Design review of the part built by this model. Coordinates are the model's own, in mm. Give positions to 0.01 mm unless a question says otherwise; leave off trailing zeros. Order: outer loops, then holes, each group sorted by start corner. A loop starts at its lowest first (then second) coordinate and runs counter-clockwise, first axis right, second up. Notation, with made-up numbers: (23, 55) -> (54, 55) arc R31 ccw to (54, 86) -> close; hole circle Ø8 at (3.25, 18). An arc over 180 degrees is marked (long way). Answer in a Markdown table with one row per item. Add a question column.
```python
from build123d import *

# Parameters (mm, degrees)
F0_R     = 10.9982
F1_DEPTH = 6.35


with BuildPart() as f1:
    # F0 (on Front) → F1 (new body)
    with BuildSketch(Plane.XZ):
        with BuildLine():
            ThreePointArc((12.7012721412, 6.542961275), (13.8852814514, 3.3662464655), (14.2875, 0))
            ThreePointArc((14.2875, 0), (9.8578957303, -10.3418831951), (-0.6842652522, -14.2711049788))
            ThreePointArc((-0.6842652522, -14.2711049788), (7.240663618, -16.8071465228), (12.8358325851, -22.965887347))
            ThreePointArc((12.8358325851, -22.965887347), (13.5200979128, -8.6947823719), (26.2213700252, -2.151821041))
            ThreePointArc((26.2213700252, -2.151821041), (18.2964411378, 0.3842204693), (12.7012721412, 6.542961275))
        make_face()
        with BuildLine():
            ThreePointArc((-14.9742166985, -21.6324620433), (-8.8154758203, -16.0372930271), (-0.6842652522, -14.2711049788))
            ThreePointArc((-0.6842652522, -14.2711049788), (-12.7012721174, -6.5429613211), (-12.0170067319, 7.7281437263))
            ThreePointArc((-12.0170067319, 7.7281437263), (-18.1757475859, 2.1329746676), (-26.3069581555, 0.366786576))
            ThreePointArc((-26.3069581555, 0.366786576), (-16.649340262, -4.0464226961), (-12.7037234832, -13.9043183991))
            ThreePointArc((-12.7037234832, -13.9043183991), (-13.283093766, -17.9317041401), (-14.9742166985, -21.6324620433))
        make_face()
        with BuildLine():
            ThreePointArc((-12.0170067319, 7.7281437263), (0.6842654078, 14.2711049713), (12.7012721412, 6.542961275))
            ThreePointArc((12.7012721412, 6.542961275), (10.9350840416, 14.6741718257), (13.4711255704, 22.5991007709))
            ThreePointArc((13.4711255704, 22.5991007709), (0.769853458, 16.0561394401), (-11.2471533267, 23.7842830843))
            ThreePointArc((-11.2471533267, 23.7842830843), (-9.4809652551, 15.6530726068), (-12.0170067319, 7.7281437263))
        make_face()
        with BuildLine():
            ThreePointArc((39.8246046975, -16.4229260161), (35.8789879186, -6.5650303131), (26.2213700252, -2.151821041))
            ThreePointArc((26.2213700252, -2.151821041), (13.5200979128, -8.6947823719), (12.8358325851, -22.965887347))
            ThreePointArc((12.8358325851, -22.965887347), (28.9033511936, -30.3082074601), (39.8246046975, -16.4229260161))
        make_face()
        with Locations((25.5371046975, -16.4229260161)):
            Circle(F0_R, mode=Mode.SUBTRACT)
        with BuildLine():
            ThreePointArc((-11.2471533267, 23.7842830843), (0.769853458, 16.0561394401), (13.4711255704, 22.5991007709))
            ThreePointArc((13.4711255704, 22.5991007709), (15.1622485029, 26.2998586742), (15.7416187857, 30.3272444152))
            ThreePointArc((15.7416187857, 30.3272444152), (-1.9121277104, 44.2125258591), (-11.2471533267, 23.7842830843))
        make_face()
        with Locations((1.4541187857, 30.3272444152)):
            Circle(F0_R, mode=Mode.SUBTRACT)
        with BuildLine():
            ThreePointArc((-0.6842652522, -14.2711049788), (9.8578957303, -10.3418831951), (14.2875, 0))
            ThreePointArc((14.2875, 0), (13.8852814514, 3.3662464655), (12.7012721412, 6.542961275))
            ThreePointArc((12.7012721412, 6.542961275), (0.6842654078, 14.2711049713), (-12.0170067319, 7.7281437263))
            ThreePointArc((-12.0170067319, 7.7281437263), (-12.7012721174, -6.5429613211), (-0.6842652522, -14.2711049788))
        make_face()
        Circle(F0_R, mode=Mode.SUBTRACT)
        with BuildLine():
            ThreePointArc((-26.3069581555, 0.366786576), (-39.6924955955, -20.44727973), (-14.9742166985, -21.6324620433))
            ThreePointArc((-14.9742166985, -21.6324620433), (-13.283093766, -17.9317041401), (-12.7037234832, -13.9043183991))
            ThreePointArc((-12.7037234832, -13.9043183991), (-16.649340262, -4.0464226961), (-26.3069581555, 0.366786576))
        make_face()
        with Locations((-26.9912234832, -13.9043183991)):
            Circle(F0_R, mode=Mode.SUBTRACT)
    extrude(amount=F1_DEPTH)


solid = f1.part
```
1) Mouldability with a two-part tool opening along Z and no side actions: class faces 1 (the face through (-39.88, -3.13, -20.07)), 2 (the face through (-7, 0, -10)), 3 (the face through (-16.5, -3.1, -10.6)) as +Z half, -Z half, draft (parallel to the pull), parting line (faces both ways), or undercut.
2) Clearance check with a flat-ended pin moving along its axis: P1, Ø2, axis at y = -3.5, z = 23, coming from the -X side. State where the tip first meets the part, or that it passes through.
3) For L1, parallel to X at y = -1.75, z = 30; L2, parallel to Z at x = 5, y = -4.5; L3, parallel to X at y = -0.75, z = -18, list the stretches that pass through material, from the lowest coordinate up.
4) Add section A-A, the plane z = -1. Write out the cut boundary in (x, y).
5) Add section B-B, the plane x = -28. Write out the cut boundary in (y, z), and give its area (3 significant figures).
6) Add section D-D, the plane z = 16. Write out the cut boundary in (x, y), and give its area (3 significant figures).
7) Add section C-C, the plane y = -4. Write out the cut boundary in (x, z) (1 decimal).
Verdict:
| question | item | result |
|---|---|---|
| 1 | face 1 | parting line |
| 1 | face 2 | draft |
| 1 | face 3 | undercut |
| 2 | P1 | stops at x = -11.36 |
| 3 | L1 | x = -12.83 to -9.54, 12.45 to 15.74 |
| 3 | L2 | z = -15.61 to -9.8, 9.8 to 19.92, 40.74 to 44.17 |
| 3 | L3 | x = -40.68 to -37.2, -16.78 to -11.77, 8.86 to 14.65, 36.42 to 39.74 |
| 4 | outline | (-33.12, -6.35) -> (-10.95, -6.35) -> (-10.95, 0) -> (-33.12, 0) -> close; (10.95, -6.35) -> (20.97, -6.35) -> (20.97, 0) -> (10.95, 0) -> close |
| 5 | outline | (-6.35, -28.16) -> (0, -28.16) -> (0, -24.86) -> (-6.35, -24.86) -> close; (-6.35, -2.95) -> (0, -2.95) -> (0, 0.35) -> (-6.35, 0.35) -> close |
| 5 | area | 41.9 mm2 |
| 6 | outline | (-9.47, -6.35) -> (11.05, -6.35) -> (11.05, 0) -> (-9.47, 0) -> close |
| 6 | area | 130 mm2 |
| 7 | outline | (-26.3, 0.4) arc R14.3 ccw (long way) to (-15, -21.6) arc R16.1 cw to (12.8, -23) arc R14.3 ccw (long way) to (26.2, -2.2) arc R16.1 cw to (13.5, 22.6) arc R14.3 ccw (long way) to (-11.2, 23.8) arc R16.1 cw to start; hole circle Ø22 at (-27, -13.9); hole circle Ø22 at (0, 0); hole circle Ø22 at (1.5, 30.3); hole circle Ø22 at (25.5, -16.4) |
